Geometry: see drawing. Coordinates: mm, zero at the bounding-box minimum. A direction names the side the tool comes from. Give positions to 0.01 mm unless a question says otherwise; leave off trailing zeros. Loops run counter-clockwise (first coordinate to the right, second up) from the corner with the lowest first, then second, coordinate; pieces in that order, holes last. Notation, with made-up numbers: M -32.75,27.25 L 0.25,27.25 A16 ccw 0.25,48.25 Z; hole C 44,-16.75 d4. An arc over 180 degrees is marked long. Put each result on its own line as item: value.
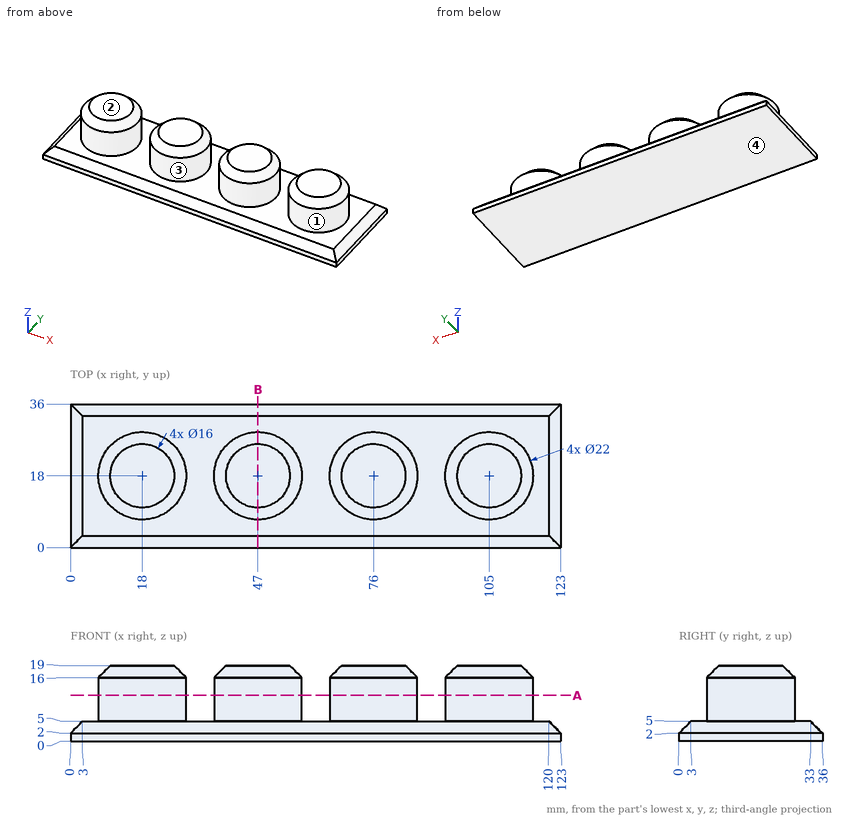
Item 1: Section B-B on x = 47. Output: boundary loops of the cut face in (y, z), then the cut area to 3 significant figures.
Output values:
outline: M 0,0 L 36,0 L 36,2 L 33,5 L 29,5 L 29,16 L 26,19 L 10,19 L 7,16 L 7,5 L 3,5 L 0,2 Z
area: 470 mm²
Item 2: Pin query (flat end, axial travel): pin 1 Ø3 at (x, z) = (27.5, 8.5) entering from +Y; pin 2 Ø8 at (y, z) = (24.5, 15) entering from +X; pin 3 Ø3 at (x, z) = (20, 2.5) entering from +Y; pin 4 Ø8 at (x, y) = (91, 27) entering from +Z. Return the tip coordinate at first contact, or that it passes through.
Output values:
pin 1: y = 25.55
pin 2: x = 115.71
pin 3: y = 36
pin 4: z = 5
Item 3: Set-up query: the marked faces 3 and 4. Return all of +Z, -Z, +X, -X, +Y, -Y with unobstructed straight access to the full face (end or side cutting, diameter ignored); none if empty.
Output values:
face 3: +Z
face 4: -Z, +X, -X, +Y, -Y
Item 4: Section A-A on z = 11.5. Output: boundary loops of the cut face in (x, y).
Output values:
outline: C 18,18 d22; C 47,18 d22; C 76,18 d22; C 105,18 d22
Item 5: Line query: probe 1 along X at (y, z) = (17.5, 13); probe 2 along X at (y, z) = (17.5, 18); probe 3 along Z at (x, y) = (92, 22). Output: solid intervals per line, ascending. Write a range as [from, to].
Output values:
probe 1: [7.01, 28.99], [36.01, 57.99], [65.01, 86.99], [94.01, 115.99]
probe 2: [9.01, 26.99], [38.01, 55.99], [67.01, 84.99], [96.01, 113.99]
probe 3: [0, 5]
Item 6: Mould query, pull axis X, two halves, no side actions, for the marked faces 1 and 2. Classes: pulls with the +X half, pulls with the -X half, needs draft (parallel to the pull), parting line crosses it, or undercut.
Output values:
face 1: undercut
face 2: needs draft
